```python
from build123d import *

# Parameters (mm, degrees)
SKETCH_1_W          = 10.7
SKETCH_1_H          = 5.3
EXTRUDE_1_DEPTH     = 6.4
SKETCH_2_W          = 9.9
SKETCH_2_H          = 4.5
SKETCH_2_R          = 0.4
CUT_EXTRUDE_1_DEPTH = 5
SKETCH_3_W          = 12.899416502
SKETCH_3_H          = 0.501475964
CUT_EXTRUDE_2_DEPTH = 5
SKETCH_4_R          = 0.4
EXTRUDE_2_DEPTH     = 8


with BuildPart() as part:
    # Эскиз1 → Вытянуть1 (new body)
    with BuildSketch(Plane.XY):
        Rectangle(SKETCH_1_W, SKETCH_1_H)
    extrude(amount=EXTRUDE_1_DEPTH)

    # Эскиз2 → Вырез-Вытянуть1 (cut)
    with BuildSketch(Plane.XY.offset(6.4)):
        Rectangle(SKETCH_2_W, SKETCH_2_H)
        with Locations((-1.27, 0)):
            Circle(SKETCH_2_R, mode=Mode.SUBTRACT)
        with Locations((1.27, 0)):
            Circle(SKETCH_2_R, mode=Mode.SUBTRACT)
        with Locations((-3.81, 0)):
            Circle(SKETCH_2_R, mode=Mode.SUBTRACT)
        with Locations(Location((3.81, 0, 0), (0, 0, 180))):
            Circle(SKETCH_2_R, mode=Mode.SUBTRACT)
    extrude(amount=-CUT_EXTRUDE_1_DEPTH, mode=Mode.SUBTRACT)

    # Эскиз3 → Вырез-Вытянуть2 (cut)
    with BuildSketch(Plane.XY.offset(6.4)):
        with Locations((-0.066925705, -2.002104797)):
            Rectangle(SKETCH_3_W, SKETCH_3_H)
    extrude(amount=-CUT_EXTRUDE_2_DEPTH, mode=Mode.SUBTRACT)

    # Эскиз4 → Вытянуть2 (add)
    with BuildSketch(Plane.XY.offset(6.4)):
        with Locations((-1.27, 0)):
            Circle(SKETCH_4_R)
        with Locations((1.27, 0)):
            Circle(SKETCH_4_R)
        with Locations((-3.81, 0)):
            Circle(SKETCH_4_R)
        with Locations(Location((3.81, 0, 0), (0, 0, 180))):
            Circle(SKETCH_4_R)
    extrude(amount=-EXTRUDE_2_DEPTH)


solid = part.part
```
CAD build for the part. Positions are in the model's coordinates, mm. A direction names the side the tool comes from. Round coordinates to 2 decimals unless told otherwise and drop trailing zeros. Write each loop counter-clockwise with the first axis right and the second up, starting at its lowest first coordinate (ties: lowest second). Pieces come first, ordered by that corner, then holes. Notation, with made-up numbers: (23, -11.75) -> (27, -11.75) arc R28 cw to (27, 24.25) -> close; hole circle Ø2 at (51, 23.5). An arc over 180 degrees is marked (long way). Answer in a Markdown table with one row per item. Add a question column.
Item 1: Saw through at D-D, the plane x = 0. Write the cut outline in (y, z), then the cut area to 3 significant figures.
Item 2: Saw through at A-A, the plane z = 5.75. Write the cut outline in (x, y), then the cut area to 3 significant figures.
Item 3: Saw through at B-B, the plane x = 3.81. Write the cut outline in (y, z).
Item 4: Drop a flat-ended pin along its axis: pin 1 Ø1.4 at (x, y) = (2.5, 0) entering from +Z. Give the stop position or say it passes through.
Item 5: Which spindle directions (+Z, -Z, +X, -X, +Y, -Y) get a long thin tool onto all of the face, cutting with end or side? Do faces 5 (the face through (0, 2.25, 4)), 6 (the face through (5.35, 0, 3)). Say none if no direction does.
Item 6: Drill centre lines: line 1 (X direction, y = 0.05, z = 1.5); line 2 (Y direction, x = 2, z = 3); line 3 (X direction, y = -1, z = 3.25). Where is each one in solid material? Low to high. Write a range as from..to.
Item 7: Saw through at C-C, the plane y = 0.65. Write the cut outline in (x, z), then the cut area to 3 significant figures.
Item 8: Mould opens along X. For faces 1 (the face through (0, 0, 1.4)), 2 (the face through (0, -2.253, 4)), 3 (the face through (4.95, 0, 4)), 4 (the face through (-5.35, 0, 3)) say: pulls with the +X half, pulls with the -X half, needs draft (parallel to the pull), parting line crosses it, or undercut.
Findings below:
| question | item | result |
|---|---|---|
| 1 | outline | (-2.65, 0) -> (2.65, 0) -> (2.65, 6.4) -> (2.25, 6.4) -> (2.25, 1.4) -> (-2.25, 1.4) -> (-2.25, 6.4) -> (-2.65, 6.4) -> close |
| 1 | area | 11.4 mm^2 |
| 2 | outline | (-5.35, -2.65) -> (5.35, -2.65) -> (5.35, -2.25) -> (-5.35, -2.25) -> close; (-5.35, -1.75) -> (-4.95, -1.75) -> (-4.95, 2.25) -> (4.95, 2.25) -> (4.95, -1.75) -> (5.35, -1.75) -> (5.35, 2.65) -> (-5.35, 2.65) -> close; circle Ø0.8 at (-3.81, 0); circle Ø0.8 at (-1.27, 0); circle Ø0.8 at (1.27, 0); circle Ø0.8 at (3.81, 0) |
| 2 | area | 13.7 mm^2 |
| 3 | outline | (-2.65, 0) -> (-0.4, 0) -> (-0.4, -1.6) -> (0.4, -1.6) -> (0.4, 0) -> (2.65, 0) -> (2.65, 6.4) -> (2.25, 6.4) -> (2.25, 1.4) -> (0.4, 1.4) -> (0.4, 6.4) -> (-0.4, 6.4) -> (-0.4, 1.4) -> (-2.25, 1.4) -> (-2.25, 6.4) -> (-2.65, 6.4) -> close |
| 4 | pin 1 | stops at z = 1.4 |
| 5 | face 5 | +Z |
| 5 | face 6 | +Z, -Z, +X, +Y, -Y |
| 6 | line 1 | x = -5.35..-4.95, -4.21..-3.41, -1.67..-0.87, 0.87..1.67, 3.41..4.21, 4.95..5.35 |
| 6 | line 2 | y = -2.65..-2.25, 2.25..2.65 |
| 6 | line 3 | x = -5.35..-4.95, 4.95..5.35 |
| 7 | outline | (-5.35, 0) -> (5.35, 0) -> (5.35, 6.4) -> (4.95, 6.4) -> (4.95, 1.4) -> (-4.95, 1.4) -> (-4.95, 6.4) -> (-5.35, 6.4) -> close |
| 7 | area | 19.0 mm^2 |
| 8 | face 1 | undercut |
| 8 | face 2 | needs draft |
| 8 | face 3 | undercut |
| 8 | face 4 | pulls with the -X half |
